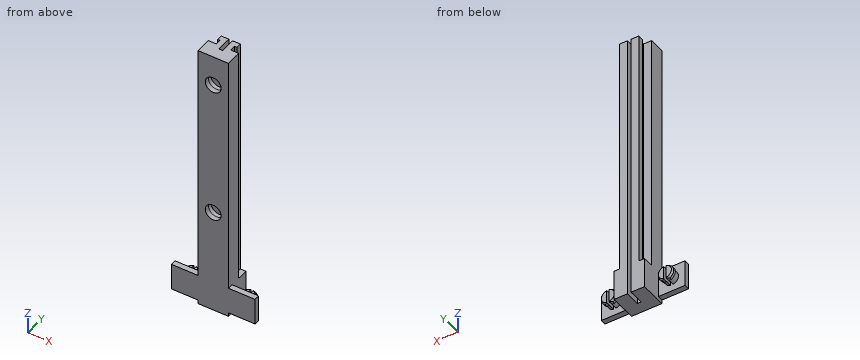
```python
from build123d import *

# Parameters (mm, degrees)
SKETCH1_W             = 12.7
SKETCH1_H             = 114.3
BOSS_EXTRUDE1_DEPTH   = 11.1125
SKETCH2_W             = 1.5875
SKETCH2_H             = 6.35
CUT_EXTRUDE1_DEPTH    = 115.3
CUT_EXTRUDE2_DEPTH    = 101.6
SKETCH4_W             = 11.1125
SKETCH4_H             = 11.1125
BOSS_EXTRUDE2_DEPTH   = 2.286
BOSS_EXTRUDE3_DEPTH   = 2.54
BOSS_EXTRUDE5_DEPTH   = 1.778
CHAMFER1_SIZE         = 0.79375
CHAMFER1_SIZE2        = 0.458271776
CHAMFER1_PART_2_SIZE  = 0.79375
CHAMFER1_PART_2_SIZE2 = 0.458271776
CHAMFER1_PART_3_SIZE  = 0.79375
CHAMFER1_PART_3_SIZE2 = 0.458271776
CHAMFER1_PART_4_SIZE  = 0.79375
CHAMFER1_PART_4_SIZE2 = 0.458271776
SKETCH7_R             = 3.302
CUT_EXTRUDE3_DEPTH    = 2.032
SKETCH8_R             = 3.556
CUT_EXTRUDE4_DEPTH    = 1.905


with BuildPart() as part:
    # Sketch1 → Boss-Extrude1 (new body)
    with BuildSketch(Plane(origin=(0, 0, 0), x_dir=(1, 0, 0), z_dir=(0, 1, 0))):
        with Locations((6.35, -57.15)):
            Rectangle(SKETCH1_W, SKETCH1_H)
    extrude(amount=BOSS_EXTRUDE1_DEPTH)

    # Sketch2 → Cut-Extrude1 (cut, through all)
    with BuildSketch(Plane.XY.offset(114.3)):
        with Locations((6.35, 7.9375)):
            Rectangle(SKETCH2_W, SKETCH2_H)
    extrude(amount=-CUT_EXTRUDE1_DEPTH, mode=Mode.SUBTRACT)

    # Sketch3 → Cut-Extrude2 (cut)
    with BuildSketch(Plane.XY.offset(114.3)):
        Polygon((2.3622, 11.1125), (2.3622, 8.9027), (3.34645, 8.9027), (3.34645, 6.5405), (0, 6.5405), (0, 11.1125), align=None)
        Polygon((10.3378, 11.1125), (10.3378, 8.9027), (9.35355, 8.9027), (9.35355, 6.5405), (12.7, 6.5405), (12.7, 11.1125), align=None)
    extrude(amount=-CUT_EXTRUDE2_DEPTH, mode=Mode.SUBTRACT)

    # Sketch4 → Boss-Extrude2 (add)
    with BuildSketch(Plane.XZ):
        with Locations((-5.55625, 7.14375)):
            Rectangle(SKETCH4_W, SKETCH4_H)
        with Locations((18.25625, 7.14375)):
            Rectangle(SKETCH4_W, SKETCH4_H)
    extrude(amount=-BOSS_EXTRUDE2_DEPTH)

    # Sketch5 → Boss-Extrude3 (add)
    with BuildSketch(Plane(origin=(0, 2.286, 0), x_dir=(1, 0, 0), z_dir=(0, 1, 0))):
        with BuildLine():
            Line((18.76425, -4.396319928), (18.76425, -9.891180072))
            ThreePointArc((18.76425, -9.891180072), (21.05025, -7.14375), (18.76425, -4.396319928))
        make_face()
        with BuildLine():
            Line((-6.06425, -4.34975), (-6.06425, -9.93775))
            ThreePointArc((-6.06425, -9.93775), (-8.396056331, -7.14375), (-6.06425, -4.34975))
        make_face()
        with BuildLine():
            Line((17.74825, -4.396319928), (17.74825, -9.891180072))
            ThreePointArc((17.74825, -9.891180072), (15.46225, -7.14375), (17.74825, -4.396319928))
        make_face()
        with BuildLine():
            Line((-5.04825, -4.34975), (-5.04825, -9.93775))
            ThreePointArc((-5.04825, -9.93775), (-2.716443669, -7.14375), (-5.04825, -4.34975))
        make_face()
    extrude(amount=BOSS_EXTRUDE3_DEPTH)

    # Sketch6 → Boss-Extrude5 (add)
    with BuildSketch(Plane(origin=(0, 4.826, 0), x_dir=(1, 0, 0), z_dir=(0, 1, 0))):
        with BuildLine():
            Line((-7.064291445, -4.34975), (-6.06425, -4.34975))
            Line((-6.06425, -4.34975), (-6.06425, -9.93775))
            Line((-6.06425, -9.93775), (-7.064291445, -9.93775))
            ThreePointArc((-7.064291445, -9.93775), (-8.73125, -7.14375), (-7.064291445, -4.34975))
        make_face()
        with BuildLine():
            Line((-4.048208555, -4.34975), (-5.04825, -4.34975))
            Line((-5.04825, -4.34975), (-5.04825, -9.93775))
            Line((-5.04825, -9.93775), (-4.048208555, -9.93775))
            ThreePointArc((-4.048208555, -9.93775), (-2.38125, -7.14375), (-4.048208555, -4.34975))
        make_face()
        with BuildLine():
            Line((16.664944561, -4.396319928), (17.74825, -4.396319928))
            Line((17.74825, -4.396319928), (17.74825, -9.891180072))
            Line((17.74825, -9.891180072), (16.664944561, -9.891180072))
            ThreePointArc((16.664944561, -9.891180072), (15.08125, -7.14375), (16.664944561, -4.396319928))
        make_face()
        with BuildLine():
            Line((19.847555439, -4.396319928), (18.76425, -4.396319928))
            Line((18.76425, -4.396319928), (18.76425, -9.891180072))
            Line((18.76425, -9.891180072), (19.847555439, -9.891180072))
            ThreePointArc((19.847555439, -9.891180072), (21.43125, -7.14375), (19.847555439, -4.396319928))
        make_face()
    extrude(amount=BOSS_EXTRUDE5_DEPTH)

    # Chamfer1
    chamfer1_edges = [part.edges().sort_by_distance(p)[0] for p in [
        (21.43125, 6.604, 7.14375),
    ]]
    chamfer1_side = [part.faces().sort_by_distance(p)[0] for p in [
        (21.43125, 5.715, 7.14375),
    ]]
    chamfer(chamfer1_edges, length=CHAMFER1_SIZE, length2=CHAMFER1_SIZE2, reference=chamfer1_side[0])

    # Chamfer1 part 2
    chamfer1_part_2_edges = [part.edges().sort_by_distance(p)[0] for p in [
        (15.08125, 6.604, 7.14375),
    ]]
    chamfer1_part_2_side = [part.faces().sort_by_distance(p)[0] for p in [
        (15.08125, 5.715, 7.14375),
    ]]
    chamfer(chamfer1_part_2_edges, length=CHAMFER1_PART_2_SIZE, length2=CHAMFER1_PART_2_SIZE2, reference=chamfer1_part_2_side[0])

    # Chamfer1 part 3
    chamfer1_part_3_edges = [part.edges().sort_by_distance(p)[0] for p in [
        (-2.38125, 6.604, 7.14375),
    ]]
    chamfer1_part_3_side = [part.faces().sort_by_distance(p)[0] for p in [
        (-2.38125, 5.715, 7.14375),
    ]]
    chamfer(chamfer1_part_3_edges, length=CHAMFER1_PART_3_SIZE, length2=CHAMFER1_PART_3_SIZE2, reference=chamfer1_part_3_side[0])

    # Chamfer1 part 4
    chamfer1_part_4_edges = [part.edges().sort_by_distance(p)[0] for p in [
        (-8.73125, 6.604, 7.14375),
    ]]
    chamfer1_part_4_side = [part.faces().sort_by_distance(p)[0] for p in [
        (-8.73125, 5.715, 7.14375),
    ]]
    chamfer(chamfer1_part_4_edges, length=CHAMFER1_PART_4_SIZE, length2=CHAMFER1_PART_4_SIZE2, reference=chamfer1_part_4_side[0])

    # Sketch7 → Cut-Extrude3 (cut)
    with BuildSketch(Plane.XZ):
        with Locations((6.35, 101.6)):
            Circle(SKETCH7_R)
        with Locations((6.35, 44.014136)):
            Circle(SKETCH7_R)
    extrude(amount=-CUT_EXTRUDE3_DEPTH, mode=Mode.SUBTRACT)

    # Sketch8 → Cut-Extrude4 (cut)
    with BuildSketch(Plane.XZ.offset(-2.032)):
        with Locations((6.35, 101.6)):
            Circle(SKETCH8_R)
        with Locations((6.35, 44.014136)):
            Circle(SKETCH8_R)
    extrude(amount=-CUT_EXTRUDE4_DEPTH, mode=Mode.SUBTRACT)


solid = part.part
```
Model file for the job. Use its own axes, mm. Coordinates: 2 decimals unless noted, no trailing zeros. Write each loop counter-clockwise with the first axis right and the second up, starting at its lowest first coordinate (ties: lowest second). Pieces come first, ordered by that corner, then holes. Notation, with made-up numbers: (6.25, 58.25) - (39.25, 58.25) arc R28 cw to (39.25, 90.25) - close; hole circle Ø6 at (-39, -26). An arc over 180 degrees is marked (long way). One line per question, with ' | ' between items. Start each with the question number.
Q1. Drill centre lines: line 1 (Z direction, x = 6.35, y = 2.8); line 2 (Z direction, x = 6.35, y = 0.95); line 3 (Y direction, x = 3, z = 30.5). Where is each one in solid material? Low to high. Write a range as [from, to].
Q2. Pin check, flat tips, straight feed: pin 1 (5 mm diameter, centred on x = -5, y = 10, fed in from -Z); pin 2 (0.5 mm diameter, centred on x = -5, y = 6, fed in from +Z); pin 3 (1.7 mm diameter, centred on x = 11.5, z = 56.5, fed in from +Y); pin 4 (1.3 mm diameter, centred on y = 5, z = 8, fed in from +X). Stop position of each tip, or through.
Q3. Cut at A-A, the plane z = 79. List the corners of the cut face in (x, y).
Q4. Cut at B-B, the plane z = 101.6. List the corners of the cut face in (x, y), then the cut area to 3 significant figures.
Answer below:
1) line 1: [0, 40.46], [47.57, 98.04], [105.16, 114.3] | line 2: [0, 40.71], [47.32, 98.3], [104.9, 114.3] | line 3: [0, 6.54], [8.9, 11.11]
2) pin 1: through | pin 2: z = 9.94 | pin 3: y = 6.54 | pin 4: x = 21.42
3) outline: (0, 0) - (12.7, 0) - (12.7, 6.54) - (9.35, 6.54) - (9.35, 8.9) - (10.34, 8.9) - (10.34, 11.11) - (7.14, 11.11) - (7.14, 4.76) - (5.56, 4.76) - (5.56, 11.11) - (2.36, 11.11) - (2.36, 8.9) - (3.35, 8.9) - (3.35, 6.54) - (0, 6.54) - close
4) outline: (0, 0) - (3.05, 0) - (3.05, 2.03) - (2.79, 2.03) - (2.79, 3.94) - (9.91, 3.94) - (9.91, 2.03) - (9.65, 2.03) - (9.65, 0) - (12.7, 0) - (12.7, 6.54) - (9.35, 6.54) - (9.35, 8.9) - (10.34, 8.9) - (10.34, 11.11) - (7.14, 11.11) - (7.14, 4.76) - (5.56, 4.76) - (5.56, 11.11) - (2.36, 11.11) - (2.36, 8.9) - (3.35, 8.9) - (3.35, 6.54) - (0, 6.54) - close | area: 77.8 mm^2
